from build123d import *

# Parameters (mm, degrees)
F1_DEPTH = 38.1
F2_R     = 1.5875
F3_DEPTH = 17.4762


with BuildPart() as f1:
    # F0 (on Front) → F1 (new body)
    with BuildSketch(Plane.XZ):
        Polygon((9.91235, 17.4752), (-15.48765, 17.4752), (-15.48765, 0), (-13.90015, 0), (-13.90015, 15.8877), (8.32485, 15.8877), (8.32485, 11.1252), (9.91235, 11.1252), align=None)
    extrude(amount=-F1_DEPTH)

    # F2 (on face) → F3 (cut, through all)
    with BuildSketch(Plane.XY.offset(17.4752)):
        with BuildLine():
            Line((-1.49225, 3.2258), (0.79375, 3.2258))
            Line((0.79375, 3.2258), (0.79375, 5.5118))
            ThreePointArc((0.79375, 5.5118), (-0.822696, 4.842246), (-1.49225, 3.2258))
        make_face()
        with BuildLine():
            Line((0.79375, 5.5118), (0.79375, 3.2258))
            Line((0.79375, 3.2258), (3.07975, 3.2258))
            ThreePointArc((3.07975, 3.2258), (2.410196, 4.842246), (0.79375, 5.5118))
        make_face()
        with BuildLine():
            Line((3.07975, 3.2258), (0.79375, 3.2258))
            Line((0.79375, 3.2258), (-1.49225, 3.2258))
            ThreePointArc((-1.49225, 3.2258), (0.79375, 0.9398), (3.07975, 3.2258))
        make_face()
        with BuildLine():
            ThreePointArc((-1.49225, 34.8742), (-0.822696, 33.257754), (0.79375, 32.5882))
            Line((0.79375, 32.5882), (0.79375, 34.8742))
            Line((0.79375, 34.8742), (-1.49225, 34.8742))
        make_face()
        with BuildLine():
            Line((0.79375, 34.8742), (0.79375, 32.5882))
            ThreePointArc((0.79375, 32.5882), (2.410196, 33.257754), (3.07975, 34.8742))
            Line((3.07975, 34.8742), (0.79375, 34.8742))
        make_face()
        with BuildLine():
            ThreePointArc((0.79375, 21.802591), (0.38735, 19.05), (0.79375, 16.297409))
            Line((0.79375, 16.297409), (0.79375, 21.802591))
        make_face()
        with BuildLine():
            Line((0.79375, 21.802591), (0.79375, 16.297409))
            ThreePointArc((0.79375, 16.297409), (11.303565, 9.627148), (19.43735, 19.05))
            ThreePointArc((19.43735, 19.05), (11.303565, 28.472852), (0.79375, 21.802591))
        make_face()
        with BuildLine():
            Line((-1.49225, 34.8742), (0.79375, 34.8742))
            Line((0.79375, 34.8742), (3.07975, 34.8742))
            ThreePointArc((3.07975, 34.8742), (0.79375, 37.1602), (-1.49225, 34.8742))
        make_face()
        with Locations((-9.13765, 19.05)):
            Circle(F2_R)
    extrude(amount=-F3_DEPTH, mode=Mode.SUBTRACT)


solid = f1.part
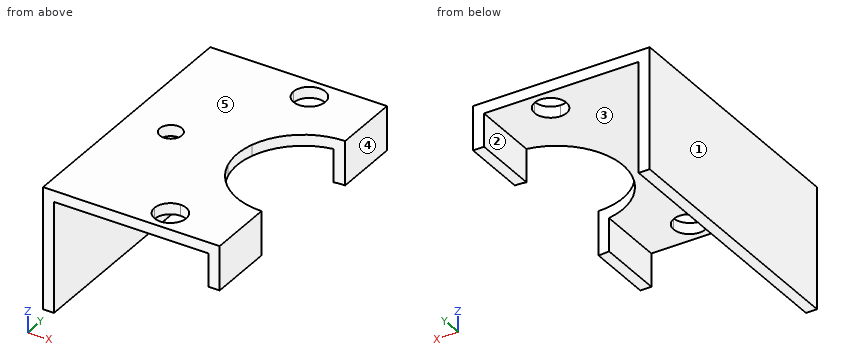
Source: CAD feature listing. Evaluate the final solid. Frame: model axes, mm. Face numbers are marked on the shaded views. A direction names the side the tool comes from. Coordinates: 2 decimals unless noted, no trailing zeros. Write each loop counter-clockwise with the first axis right and the second up, starting at its lowest first coordinate (ties: lowest second). Pieces come first, ordered by that corner, then holes. Notation, with made-up numbers: M 47.5,-11.5 L 62.5,-11.5 A23 cw 62.5,15.5 Z; hole C 19,88 d8. An arc over 180 degrees is marked long. Use a Markdown table: item, result.
1) Section B-B, the plane x = 5.25. Output: boundary loops of the cut face in (y, z).
Conclusion:
| item | result |
|---|---|
| outline | M 0,15.89 L 10.74,15.89 L 10.74,17.48 L 0,17.48 Z; M 27.36,15.89 L 38.1,15.89 L 38.1,17.48 L 27.36,17.48 Z |
2) Section D-D, the plane y = 27.5. Output: boundary loops of the cut face in (x, z), then the cut area to 3 significant figures.
Conclusion:
| item | result |
|---|---|
| outline | M -15.49,0 L -13.9,0 L -13.9,15.89 L 5.52,15.89 L 5.52,17.48 L -15.49,17.48 Z |
| area | 58.6 mm^2 |
3) Section C-C, the plane z = 7.75. Output: boundary loops of the cut face in (x, y), then the cut area to 3 significant figures.
Conclusion:
| item | result |
|---|---|
| outline | M -15.49,0 L -13.9,0 L -13.9,38.1 L -15.49,38.1 Z |
| area | 60.5 mm^2 |
4) First-contact query: pin 1 Ø5 at (x, y) = (-9, 6.5) entering from -Z; pin 2 Ø5 at (y, z) = (19.5, 7.5) entering from +X; pin 3 Ø1.3 at (x, y) = (9.5, 6) entering from -Z; pin 4 Ø10 at (y, z) = (28, 11) entering from +X. Flat tips, straight axial feed; report the tip coordinate or a pass-through.
Conclusion:
| item | result |
|---|---|
| pin 1 | stops at z = 15.89 |
| pin 2 | stops at x = -13.9 |
| pin 3 | stops at z = 11.13 |
| pin 4 | stops at x = 9.91 |
5) Reachability of the marked faces 1 and 2 from +Z, -Z, +X, -X, +Y, -Y: full face, straight path, thin tool, end or side. Return the list, or none.
Conclusion:
| item | result |
|---|---|
| face 1 | +Z, -Z, -X, +Y, -Y |
| face 2 | -Z, +Y, -Y |
6) Section A-A, the plane y = 19.05. Output: boundary loops of the cut face in (x, z).
Conclusion:
| item | result |
|---|---|
| outline | M -15.49,0 L -13.9,0 L -13.9,15.89 L -10.73,15.89 L -10.73,17.48 L -15.49,17.48 Z; M -7.55,15.89 L 0.39,15.89 L 0.39,17.48 L -7.55,17.48 Z |
7) Ray query, L1, parallel to X at y = 8.5, z = 13.75; L2, parallel to Y at x = -0.25, z = 16; L3, parallel to Z at x = -0.75, y = 17. Return the intervals inside material, ascending.
Conclusion:
| item | result |
|---|---|
| L1 | x = -15.49 to -13.9, 8.32 to 9.91 |
| L2 | y = 0 to 1.19, 5.26 to 32.84, 36.91 to 38.1 |
| L3 | z = 15.89 to 17.48 |
8) Mould query, pull axis X, two halves, no side actions, for the marked faces 3, 4 and 5. Classes: pulls with the +X half, pulls with the -X half, needs draft (parallel to the pull), parting line crosses it, or undercut.
Conclusion:
| item | result |
|---|---|
| face 3 | undercut |
| face 4 | pulls with the +X half |
| face 5 | needs draft |
